```python
from build123d import *

# Parameters (mm, degrees)
F3_W = 3.1359323766
F3_H = 60.3541191667


with BuildPart() as f2:
    # F0 (on Right) → F2 (revolve)
    with BuildSketch(Plane.YZ):
        Polygon((0, 1.7982171848), (0, 63.0117803812), (-17.3947568983, 63.0117803812), (-17.3947568983, 57.600159198), (-6.2708631158, 57.600159198), (-6.2708631158, 40.162704885), (-6.2708631158, 5.5884346366), (-19.9502557516, 5.5884346366), (-19.9502557516, 1.7982171848), align=None)
    revolve(axis=Axis((0, -6.3099395484, 0), (0, -1, 0)))

    # F3 (on Right) → F4 (revolve, cut)
    with BuildSketch(Plane.YZ):
        with Locations((-1.5679661883, 30.1770595834)):
            Rectangle(F3_W, F3_H)
    revolve(axis=Axis((0, -6.3099395484, 0), (0, -1, 0)), mode=Mode.SUBTRACT)


solid = f2.part
```
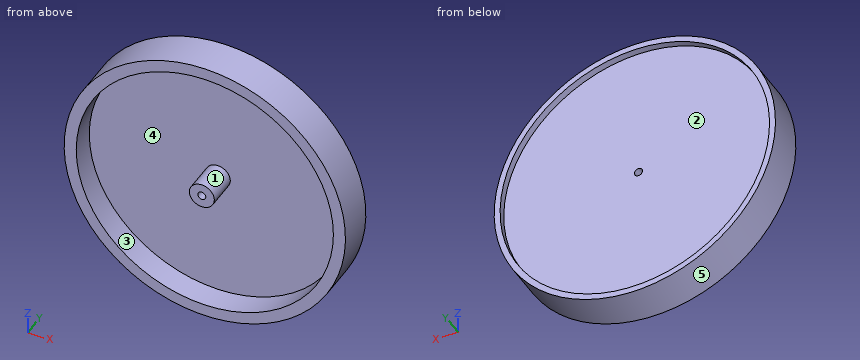
Read the model definition and answer for the solid it produces. Units are mm, in the model's axes. Face numbers are marked on the shaded views. A direction names the side the tool comes from. Give positions to 0.01 mm unless a question says otherwise; leave off trailing zeros. Write each loop counter-clockwise with the first axis right and the second up, starting at its lowest first coordinate (ties: lowest second). Pieces come first, ordered by that corner, then holes. Notation, with made-up numbers: M -23.75,33.25 L 9.25,33.25 A16 cw 9.25,53.25 Z; hole C -4.5,46.5 d9. An arc over 180 degrees is marked long. Put each result on its own line as item: value. Start each with the question number.
1. For a pull along Z with two mould halves and no side action, classify the marked faces 3, 4 and 5 as released by +Z, released by -Z, zero draft, split by the parting line, or undercut.
2. Which of the six approach directions +Z, -Z, +X, -X, +Y, -Y give full straight-line access (tool end or side, diameter ignored) to the marked faces 1 and 2?
3. The part is cut by section D-D, the plane z = 18. Give the vertices of the cut face in (x, y), and give its area (3 significant figures).
4. The part is cut by section C-C, the plane x = 0. Give the vertices of the cut face in (y, z), and give its area (3 significant figures).
5. Each of these flat-tipped pins is pushed along its axis until it touches: pin 1 Ø2 at (x, y) = (-48.5, -11) entering from -Z; pin 2 Ø10 at (y, z) = (-4, -23.5) entering from +X; pin 3 Ø6 at (x, z) = (-4.5, -14.5) entering from +Y; pin 4 Ø3 at (x, z) = (0, 0) entering from +Y. Where does it stop, or does it pass through?
6. The part is cut by section B-B, the plane y = -13.25. Give the vertices of the cut face in (x, z), and give its area (3 significant figures).
7. Consider line 1 along X through (y, z) = (-15, 0); line 2 along X through (y, z) = (-1, 0). Determine where each line is inside the solid, lowest interval first.
8. The part is cut by section A-A, the plane z = 0. Give the vertices of the cut face in (x, y), and give its area (3 significant figures).
Final values:
1. face 3: undercut
1. face 4: undercut
1. face 5: split by the parting line
2. face 1: -Y
2. face 2: +Y
3. outline: M -60.39,-17.39 L -54.72,-17.39 L -54.72,-6.27 L 54.72,-6.27 L 54.72,-17.39 L 60.39,-17.39 L 60.39,0 L 57.61,0 L 57.61,-3.14 L -57.61,-3.14 L -57.61,0 L -60.39,0 Z
3. area: 522 mm²
4. outline: M -19.95,-5.59 L -6.27,-5.59 L -6.27,-57.6 L -17.39,-57.6 L -17.39,-63.01 L 0,-63.01 L 0,-60.35 L -3.14,-60.35 L -3.14,-1.8 L -19.95,-1.8 Z; M -19.95,1.8 L -3.14,1.8 L -3.14,60.35 L 0,60.35 L 0,63.01 L -17.39,63.01 L -17.39,57.6 L -6.27,57.6 L -6.27,5.59 L -19.95,5.59 Z
4. area: 625 mm²
5. pin 1: stops at z = -41.4
5. pin 2: stops at x = 60.23
5. pin 3: stops at y = -3.14
5. pin 4: passes through
6. outline: C 0,0 d126.02; C 0,0 d11.18; hole C 0,0 d115.2; hole C 0,0 d3.6
6. area: 2,140 mm²
7. line 1: x = -63.01 to -57.6, -5.59 to -1.8, 1.8 to 5.59, 57.6 to 63.01
7. line 2: x = -63.01 to -60.35, 60.35 to 63.01
8. outline: M -63.01,-17.39 L -57.6,-17.39 L -57.6,-6.27 L -5.59,-6.27 L -5.59,-19.95 L -1.8,-19.95 L -1.8,-3.14 L -60.35,-3.14 L -60.35,0 L -63.01,0 Z; M 1.8,-19.95 L 5.59,-19.95 L 5.59,-6.27 L 57.6,-6.27 L 57.6,-17.39 L 63.01,-17.39 L 63.01,0 L 60.35,0 L 60.35,-3.14 L 1.8,-3.14 Z
8. area: 625 mm²
